```python
from build123d import *

# Parameters (mm, degrees)
SKETCH_1_R           = 13
SKETCH_1_R_2         = 11
EXTRUDE_1_DEPTH      = 4
EXTRUDE_2_DEPTH      = 1
EXTRUDE_2_DEPTH_BACK = 2.8
SKETCH_2_R           = 15
SKETCH_3_R           = 11
CUT_EXTRUDE_1_DEPTH  = 2.3
CUT_EXTRUDE_2_DEPTH  = 2


with BuildPart() as part:
    # 草图1 → 拉伸1 (new body)
    with BuildSketch(Plane.XY):
        Circle(SKETCH_1_R)
        Circle(SKETCH_1_R_2, mode=Mode.SUBTRACT)
    extrude(amount=EXTRUDE_1_DEPTH)

    # 草图2 → 拉伸2 (add, two sides: drawn at the far end of the back side and taken through both)
    with BuildSketch(Plane.XY.offset(4).offset(-EXTRUDE_2_DEPTH_BACK)):
        Circle(SKETCH_2_R)
    extrude(amount=EXTRUDE_2_DEPTH + EXTRUDE_2_DEPTH_BACK)

    # 草图3 → 切除-拉伸1 (cut)
    with BuildSketch(Plane(origin=(0, 0, 1.2), x_dir=(-1, 0, 0), z_dir=(0, 0, -1))):
        Circle(SKETCH_3_R)
    extrude(amount=-CUT_EXTRUDE_1_DEPTH, mode=Mode.SUBTRACT)

    # 草图4 → 切除-拉伸2 (cut)
    with BuildSketch(Plane(origin=(0, 0, 3.5), x_dir=(-1, 0, 0), z_dir=(0, 0, -1))):
        with BuildLine():
            Line((-8, -4.123105626), (-8, 4.123105626))
            ThreePointArc((-8, 4.123105626), (0, 9), (8, 4.123105626))
            Line((8, 4.123105626), (8, -4.123105626))
            ThreePointArc((8, -4.123105626), (0, -9), (-8, -4.123105626))
        make_face()
    extrude(amount=-CUT_EXTRUDE_2_DEPTH, mode=Mode.SUBTRACT)


solid = part.part
```
Build history of the part. All positions in model axes, mm. A direction names the side the tool comes from. Coordinates: 2 decimals unless noted, no trailing zeros. Order: outer loops, then holes, each group sorted by start corner. A loop starts at its lowest first (then second) coordinate and runs counter-clockwise, first axis right, second up. Notation, with made-up numbers: (77, 35.5) -> (90, 35.5) arc R9 ccw to (90, 47.5) -> close; hole circle Ø5 at (74, -13.75). An arc over 180 degrees is marked (long way). Answer in a Markdown table with one row per item. Add a question column.
Q1. Band-saw the part on A-A, the plane x = 0. List the corners of the cut face in (y, z).
Q2. Which spindle directions (+Z, -Z, +X, -X, +Y, -Y) get a long thin tool onto all of the face, cutting with end or side? Do faces 1 (the face through (6.5, -6.5, 5)), 2 (the face through (8.2, 0.1, 3.5)), 3 (the face through (8, 0, 4)). Say none if no direction does.
Q3. Mould opens along X. For faces 4 (the face through (-10.316, -7.91, 0.592)), 5 (the face through (0, -9, 4)), 6 (the face through (-11, 3, 0)) say: +X half, -X half, draft (parallel to the pull), parting line (faces both ways), or undercut.
Q4. Band-saw the part on D-D, the plane x = -10.5. List the corners of the cut face in (y, z), then the cut area to 3 significant figures.
Q5. Band-saw the part on B-B, the plane y = 0. List the corners of the cut face in (x, z).
Q6. Drop flat-ended pins along their axis: pin 1 (6.5 mm diameter, centred on x = -0.5, y = -4.5, fed in from -Z); pin 2 (1.6 mm diameter, centred on y = -1, z = 4, fed in from +X); pin 3 (1.5 mm diameter, centred on y = 2.5, z = 3.5, fed in from +X); pin 4 (1.5 mm diameter, centred on y = 9, z = 3, fed in from +X). Give the stop position or say it passes through.
Q7. Wall check: line 1 along Y through (x, z) = (0, 0.85); line 2 along Y through (x, z) = (0, 1.85). Give the ranges that are in metal, low to high. Write a range as [from, to].
Q8. Band-saw the part on C-C, the plane z = 2.3. List the corners of the cut face in (x, y), then the cut area to 3 significant figures.
Answers follow:
| question | item | result |
|---|---|---|
| 1 | outline | (-15, 1.2) -> (-13, 1.2) -> (-13, 0) -> (-11, 0) -> (-11, 3.5) -> (-9, 3.5) -> (-9, 5) -> (-15, 5) -> close; (9, 3.5) -> (11, 3.5) -> (11, 0) -> (13, 0) -> (13, 1.2) -> (15, 1.2) -> (15, 5) -> (9, 5) -> close |
| 2 | face 1 | +Z, +X, -X, +Y, -Y |
| 2 | face 2 | -Z |
| 2 | face 3 | +Z, -Z |
| 3 | face 4 | parting line |
| 3 | face 5 | undercut |
| 3 | face 6 | draft |
| 4 | outline | (-10.71, 1.2) -> (-7.66, 1.2) -> (-7.66, 0) -> (-3.28, 0) -> (-3.28, 3.5) -> (3.28, 3.5) -> (3.28, 0) -> (7.66, 0) -> (7.66, 1.2) -> (10.71, 1.2) -> (10.71, 5) -> (-10.71, 5) -> close |
| 4 | area | 76.9 mm^2 |
| 5 | outline | (-15, 1.2) -> (-13, 1.2) -> (-13, 0) -> (-11, 0) -> (-11, 3.5) -> (-8, 3.5) -> (-8, 5) -> (-15, 5) -> close; (8, 3.5) -> (11, 3.5) -> (11, 0) -> (13, 0) -> (13, 1.2) -> (15, 1.2) -> (15, 5) -> (8, 5) -> close |
| 6 | pin 1 | through |
| 6 | pin 2 | x = 15 |
| 6 | pin 3 | x = 14.9 |
| 6 | pin 4 | x = 12.53 |
| 7 | line 1 | [-13, -11], [11, 13] |
| 7 | line 2 | [-15, -11], [11, 15] |
| 8 | outline | circle Ø30 at (0, 0); hole circle Ø22 at (0, 0) |
| 8 | area | 327 mm^2 |
